```python
from build123d import *

# Parameters (mm, degrees)
F0_W     = 54.737
F0_H     = 40.132
F1_DEPTH = 11.684
F2_W     = 6.9596
F2_H     = 3.429
F3_DEPTH = 54.738
F5_DEPTH = 54.738
F7_DEPTH = 11.685
F9_DEPTH = 54.738
F10_R    = 0.79375


with BuildPart() as f1:
    # F0 (on Top) → F1 (new body)
    with BuildSketch(Plane.XY):
        with Locations((27.3685, 20.066)):
            Rectangle(F0_W, F0_H)
    extrude(amount=F1_DEPTH)

    # F2 (on face) → F3 (cut, through all)
    with BuildSketch(Plane.YZ.offset(54.737)):
        with Locations((31.9278, 9.9695)):
            Rectangle(F2_W, F2_H)
        with Locations((8.2042, 9.9695)):
            Rectangle(F2_W, F2_H)
    extrude(amount=-F3_DEPTH, mode=Mode.SUBTRACT)

    # F4 (on face) → F5 (cut, through all)
    with BuildSketch(Plane.YZ.offset(54.737)):
        Polygon((4.7244, 11.684), (0, 11.684), (4.7244, 11.287125), align=None)
        Polygon((35.4076, 11.287125), (40.132, 11.684), (35.4076, 11.684), align=None)
    extrude(amount=-F5_DEPTH, mode=Mode.SUBTRACT)

    # F6 (on face) → F7 (cut, through all)
    with BuildSketch(Plane.XY.offset(11.684)):
        with BuildLine():
            Line((0, 16.256), (6.3826718605, 16.256))
            ThreePointArc((6.3826718605, 16.256), (17.526, 20.066), (6.3826718605, 23.876))
            Line((6.3826718605, 23.876), (0, 23.876))
            Line((0, 23.876), (0, 16.256))
        make_face()
        with BuildLine():
            Line((54.737, 23.876), (48.3543281395, 23.876))
            ThreePointArc((48.3543281395, 23.876), (37.211, 20.066), (48.3543281395, 16.256))
            Line((48.3543281395, 16.256), (54.737, 16.256))
            Line((54.737, 16.256), (54.737, 23.876))
        make_face()
    extrude(amount=-F7_DEPTH, mode=Mode.SUBTRACT)

    # F8 (on face) → F9 (cut, through all)
    with BuildSketch(Plane(origin=(0, 0, 0), x_dir=(0, -1, 0), z_dir=(-1, 0, 0))):
        Polygon((-28.448, 11.287125), (-23.876, 11.684), (-28.448, 11.684), align=None)
        Polygon((-16.256, 11.684), (-11.684, 11.287125), (-11.684, 11.684), align=None)
    extrude(amount=-F9_DEPTH, mode=Mode.SUBTRACT)

    # F10
    f10_edges = [f1.edges().sort_by_distance(p)[0] for p in [
        (27.3685, 40.132, 11.684),
        (27.3685, 35.4076, 11.287125),
        (27.3685, 28.448, 11.287125),
        (27.3685, 11.684, 11.287125),
        (27.3685, 4.7244, 11.287125),
        (27.3685, 0, 11.684),
        (54.737, 16.256, 5.842),
        (54.737, 23.876, 5.842),
        (0, 23.876, 5.842),
        (0, 16.256, 5.842),
        (6.382672, 23.876, 5.842),
        (6.382672, 16.256, 5.842),
        (48.354328, 16.256, 5.842),
        (48.354328, 23.876, 5.842),
    ]]
    fillet(f10_edges, radius=F10_R)


solid = f1.part
```
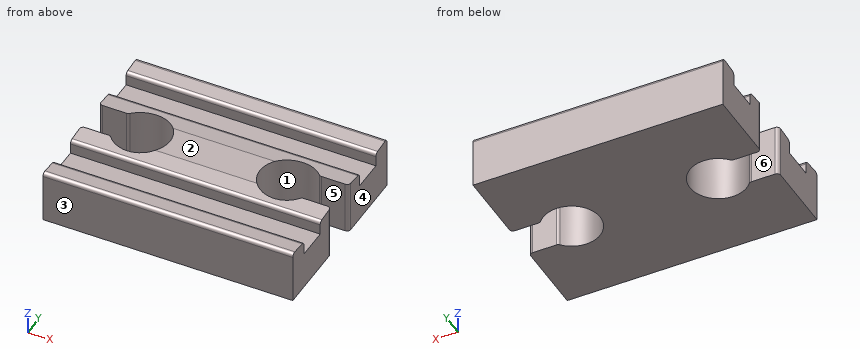
Design review of the part built by this model. Coordinates are the model's own, in mm. Face numbers are marked on the shaded views. A direction names the side the tool comes from. Give positions to 0.01 mm unless a question says otherwise; leave off trailing zeros. Loops run counter-clockwise (first coordinate to the right, second up) from the corner with the lowest first, then second, coordinate; pieces in that order, holes last. Notation, with made-up numbers: (-2, 67.25) -> (14, 67.25) arc R31 cw to (14, 97.25) -> close; hole circle Ø6 at (50.5, 20). An arc over 180 degrees is marked (long way). One line per item, written item: value.
Q1. We need section B-B on z = 6.5. Give the boundary of the cut face in (x, y), and give its area (3 significant figures).
Numbers:
outline: (0, 0) -> (54.74, 0) -> (54.74, 15.46) arc R0.79 ccw to (53.94, 16.26) -> (48.73, 16.26) arc R0.79 ccw to (48.13, 15.98) arc R6.22 cw (long way) to (48.13, 24.15) arc R0.79 ccw to (48.73, 23.88) -> (53.94, 23.88) arc R0.79 ccw to (54.74, 24.67) -> (54.74, 40.13) -> (0, 40.13) -> (0, 24.67) arc R0.79 ccw to (0.79, 23.88) -> (6.01, 23.88) arc R0.79 ccw to (6.61, 24.15) arc R6.22 cw (long way) to (6.61, 15.98) arc R0.79 ccw to (6.01, 16.26) -> (0.79, 16.26) arc R0.79 ccw to (0, 15.46) -> close
area: 1,870 mm^2
Q2. We need section A-A on x = 51.5. Give the boundary of the cut face in (y, z) (1 decimal).
Numbers:
outline: (0, 0) -> (16.3, 0) -> (16.3, 11.7) -> (12.4, 11.4) arc R0.8 ccw to (11.7, 10.6) -> (11.7, 8.3) -> (4.7, 8.3) -> (4.7, 10.6) arc R0.8 ccw to (4, 11.3) -> (0.9, 11.6) arc R0.8 ccw to (0, 10.8) -> close; (23.9, 0) -> (40.1, 0) -> (40.1, 10.8) arc R0.8 ccw to (39.3, 11.6) -> (36.1, 11.3) arc R0.8 ccw to (35.4, 10.6) -> (35.4, 8.3) -> (28.4, 8.3) -> (28.4, 10.6) arc R0.8 ccw to (27.7, 11.4) -> (23.9, 11.7) -> close
Q3. For pin 1 Ø4 at (x, y) = (28, 27) entering from +Z; pin 2 Ø7.5 at (x, y) = (40.5, 9) entering from +Z; pin 3 Ø6 at (x, y) = (23.5, 11.5) entering from +Z; pin 4 Ø2 at (x, y) = (40.5, 24) entering from +Z, all flat-tipped, find the tip position at first contact; note any pin that passes through.
Numbers:
pin 1: stops at z = 11.59
pin 2: stops at z = 11.38
pin 3: stops at z = 11.53
pin 4: passes through
Q4. Draft analysis for pull direction Y (two halves, no side actions). For the marked faces 1, 2 and 3, state which applies: pulls with the +Y half, pulls with the -Y half, needs draft (parallel to the pull), parting line crosses it, or undercut.
Numbers:
face 1: undercut
face 2: needs draft
face 3: pulls with the -Y half
Q5. Machinability: for the marked faces 4, 5 and 6, which of the approach directions +Z, -Z, +X, -X, +Y, -Y give a long, thin tool a straight path to every point of the face, cutting with its end or side? Answer none if there is none.
Numbers:
face 4: +Z, -Z, +X, +Y, -Y
face 5: +Z, -Z, +X
face 6: +Z, -Z, -X
Q6. For L1, parallel to X at y = 24, z = 8.25; L2, parallel to Y at x = 26, z = 11; L3, parallel to X at y = 15, z = 3.5, list the stretches that pass through material, from the lowest coordinate up.
Numbers:
L1: x = 0.37 to 6.43, 16.12 to 38.61, 48.3 to 54.37
L2: y = 0.02 to 4.59, 11.82 to 28.31, 35.54 to 40.11
L3: x = 0 to 7.69, 14.92 to 39.82, 47.05 to 54.74
Q7. We need section D-D on y = 8.5. Give the boundary of the cut face in (x, z) (3 decimals), and give its area (3 significant figures).
Numbers:
outline: (0, 0) -> (54.737, 0) -> (54.737, 8.255) -> (0, 8.255) -> close
area: 452 mm^2
Q8. We need section C-C on x = 22. Give the boundary of the cut face in (y, z) (1 decimal), and give its area (3 significant figures).
Numbers:
outline: (0, 0) -> (40.1, 0) -> (40.1, 10.8) arc R0.8 ccw to (39.3, 11.6) -> (36.1, 11.3) arc R0.8 ccw to (35.4, 10.6) -> (35.4, 8.3) -> (28.4, 8.3) -> (28.4, 10.6) arc R0.8 ccw to (27.7, 11.4) -> (23.9, 11.7) -> (16.3, 11.7) -> (12.4, 11.4) arc R0.8 ccw to (11.7, 10.6) -> (11.7, 8.3) -> (4.7, 8.3) -> (4.7, 10.6) arc R0.8 ccw to (4, 11.3) -> (0.9, 11.6) arc R0.8 ccw to (0, 10.8) -> close
area: 417 mm^2
